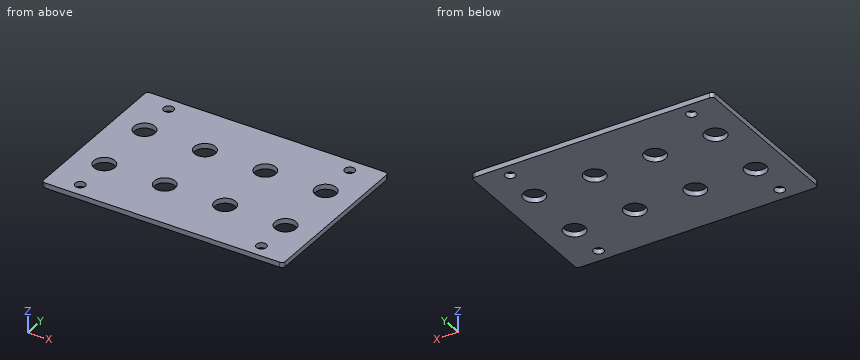
Autodesk Fusion 360 part; units mm, degrees
sketch "Sketch1" plane through (0, 0, 0) normal (0, 0, 1) x (1, 0, 0)
  circle A0 centre (9, 34.525) radius 3.95
  circle A1 centre (9, 15.475) radius 3.95
  line L0 (9, 34.525) -> (9, 15.475) construction
  circle A2 centre (9, 45.975) radius 1.5
  circle A3 centre (9, 4.025) radius 1.5
  line L1 (-1.2896, 25) -> (19.2896, 25) construction
  line L2 (9, 45.975) -> (9, 4.025) construction
  line L3 (5.7, 40.3994) -> (5.7, 10.52)
  line L4 (5.7, 10.52) -> (12.3, 10.52) construction
  line L5 (12.3, 10.52) -> (12.3, 40.3994)
  line L6 (12.3, 40.3994) -> (5.7, 40.3994) construction
  line L7 (5.05, 34.525) -> (12.95, 34.525) construction
  circle A4 centre (27, 34.525) radius 3.95
  line L8 (23.7, 40.3994) -> (23.7, 10.52)
  line L9 (30.3, 10.52) -> (30.3, 40.3994)
  circle A5 centre (27, 15.475) radius 3.95
  circle A6 centre (27, 4.025) radius 1.5
  circle A7 centre (27, 45.975) radius 1.5
  circle A8 centre (45, 34.525) radius 3.95
  line L10 (41.7, 40.3994) -> (41.7, 10.52)
  line L11 (48.3, 10.52) -> (48.3, 40.3994)
  circle A9 centre (45, 15.475) radius 3.95
  circle A10 centre (45, 4.025) radius 1.5
  circle A11 centre (45, 45.975) radius 1.5
  line L12 (0, 50) -> (72, 50)
  line L13 (72, 50) -> (72, 0)
  line L14 (72, 0) -> (0, 0)
  line L15 (0, 0) -> (0, 50)
  line L16 (27, 45.975) -> (27, 4.025) construction
  line L17 (45, 45.975) -> (45, 4.025) construction
  circle A12 centre (63, 34.525) radius 3.95
  line L18 (59.7, 40.3994) -> (59.7, 10.52)
  line L19 (66.3, 10.52) -> (66.3, 40.3994)
  circle A13 centre (63, 15.475) radius 3.95
  circle A14 centre (63, 4.025) radius 1.5
  circle A15 centre (63, 45.975) radius 1.5
  line L20 (63, 45.975) -> (63, 4.025) construction
  line L21 (36, 50) -> (36, 0) construction
  line L22 (0, 25) -> (72, 25) construction
  line L23 (9, 15.475) -> (27, 15.475) construction
  line L24 (18, 15.475) -> (18, 27.912) construction
  point P0 (9, 5.525)
  point P1 (9, 11.525)
  point P2 (27, 34.525)
  point P3 (27, 15.475)
  point P4 (45, 34.525)
  point P5 (45, 15.475)
  point P6 (63, 34.525)
  point P7 (63, 15.475)
  point P8 (45, -15.475)
  point P9 (0, -50)
  point P10 (0, -25)
  point P11 (45, -45.975)
  point P12 (45, -34.525)
  point P13 (0, 50)
  dimension "d4" = 7.9
  dimension "d5" = 7.9
  dimension "d6" = 19.05
  dimension "d7" = 6
  dimension "d8" = 3
  dimension "d9" = 0.65
  dimension "d12" = 18
  dimension "d13" = 0
  dimension "d19" = 50
  dimension "d24" = 41.95
  dimension "d34" = 9
  dimension "d35" = 9
  dimension "d36" = 9
extrude "Extrude1" add sketch "Sketch1" along normal blind 1.5 contours A0 L5 | A0 A1 L3 L5 | A0 L3 | A1 L5 | A1 L3 | A4 L9 | A4 L8 L9 A5 | A4 L8 | L9 A5 | L8 A5 | A6 | A7 | A8 L11 | A8 L10 L11 A9 | A8 L10 | L11 A9 | L10 A9 | A10 | A11 | L12 L13 L14 L15 | A12 L19 | A12 L18 L19 A13 | A12 L18 | L19 A13 | L18 A13 makes body 1
sketch "Sketch2" plane through (0, 0, 0) normal (0, 0, -1) x (1, 0, 0)
  circle A0 centre (9, -4.025) radius 1.5
  circle A1 centre (63, -4.025) radius 1.5
  arc A2 (12.3, -13.3042) -> (5.7, -13.3042) centre (9, -15.475) ccw construction
  line L0 (12.3, -13.3042) -> (12.3, -17.6458) construction
  arc A3 (5.7, -17.6458) -> (12.3, -17.6458) centre (9, -15.475) ccw construction
  line L1 (5.7, -17.6458) -> (5.7, -13.3042) construction
  line L2 (30.3, -13.3042) -> (30.3, -17.6458) construction
  arc A4 (23.7, -17.6458) -> (30.3, -17.6458) centre (27, -15.475) ccw construction
  line L3 (23.7, -17.6458) -> (23.7, -13.3042) construction
  arc A5 (30.3, -13.3042) -> (23.7, -13.3042) centre (27, -15.475) ccw construction
  circle A6 centre (63, -45.975) radius 1.5
  line L4 (48.3, -13.3042) -> (48.3, -17.6458) construction
  arc A7 (41.7, -17.6458) -> (48.3, -17.6458) centre (45, -15.475) ccw construction
  line L5 (41.7, -17.6458) -> (41.7, -13.3042) construction
  arc A8 (48.3, -13.3042) -> (41.7, -13.3042) centre (45, -15.475) ccw construction
  circle A9 centre (9, -45.975) radius 1.5
  line L6 (66.3, -13.3042) -> (66.3, -17.6458) construction
  arc A10 (59.7, -17.6458) -> (66.3, -17.6458) centre (63, -15.475) ccw construction
  line L7 (59.7, -17.6458) -> (59.7, -13.3042) construction
  arc A11 (66.3, -13.3042) -> (59.7, -13.3042) centre (63, -15.475) ccw construction
  line L8 (72, 0) -> (0, 0)
  line L9 (0, 0) -> (0, -50)
  line L10 (0, -50) -> (72, -50)
  line L11 (72, -50) -> (72, 0)
  line L12 (0.4311, -10.2537) -> (71.5689, -10.2537)
  line L13 (71.5689, -10.2537) -> (71.5689, -39.7463)
  line L14 (71.5689, -39.7463) -> (0.4311, -39.7463)
  line L15 (0.4311, -39.7463) -> (0.4311, -10.2537)
  line L16 (0, -25) -> (72, -25) construction
  line L17 (27, -45.975) -> (27, -4.025) construction
  line L18 (45, -45.975) -> (45, -4.025) construction
  line L19 (63, -45.975) -> (63, -4.025) construction
  line L20 (9, -45.975) -> (9, -4.025) construction
  line L21 (36, 0) -> (36, -50) construction
  line L22 (73.0689, -8.7537) -> (73.0689, -41.2463)
  line L23 (73.0689, -41.2463) -> (-1.0689, -41.2463)
  line L24 (-1.0689, -41.2463) -> (-1.0689, -8.7537)
  line L25 (-1.0689, -8.7537) -> (73.0689, -8.7537)
  arc A12 (12.3, -32.3542) -> (5.7, -32.3542) centre (9, -34.525) ccw
  line L26 (12.3, -32.3542) -> (12.3, -36.6958)
  arc A13 (5.7, -36.6958) -> (12.3, -36.6958) centre (9, -34.525) ccw
  line L27 (5.7, -36.6958) -> (5.7, -32.3542)
  arc A14 (66.3, -32.3542) -> (59.7, -32.3542) centre (63, -34.525) ccw
  line L28 (66.3, -32.3542) -> (66.3, -36.6958)
  arc A15 (59.7, -36.6958) -> (66.3, -36.6958) centre (63, -34.525) ccw
  line L29 (59.7, -36.6958) -> (59.7, -32.3542)
  arc A16 (30.3, -32.3542) -> (23.7, -32.3542) centre (27, -34.525) ccw
  line L30 (30.3, -32.3542) -> (30.3, -36.6958)
  arc A17 (23.7, -36.6958) -> (30.3, -36.6958) centre (27, -34.525) ccw
  line L31 (23.7, -36.6958) -> (23.7, -32.3542)
  arc A18 (48.3, -32.3542) -> (41.7, -32.3542) centre (45, -34.525) ccw
  line L32 (48.3, -32.3542) -> (48.3, -36.6958)
  arc A19 (41.7, -36.6958) -> (48.3, -36.6958) centre (45, -34.525) ccw
  line L33 (41.7, -36.6958) -> (41.7, -32.3542)
  dimension "d18" = -1.5
sketch "Sketch3" plane through (0, 0, 0) normal (0, 0, 1) x (1, 0, 0)
  line L0 (0, 50) -> (72, 50)
  line L1 (72, 50) -> (72, 0)
  line L2 (72, 0) -> (0, 0)
  line L3 (0, 0) -> (0, 50)
  circle A0 centre (9, 45.975) radius 1.5
  circle A1 centre (9, 4.025) radius 1.5
  circle A2 centre (9, 34.525) radius 3.15
  circle A3 centre (9, 15.475) radius 3.15
  circle A4 centre (27, 34.525) radius 3.15
  circle A5 centre (27, 45.975) radius 1.5
  circle A6 centre (27, 15.475) radius 3.15
  circle A7 centre (27, 4.025) radius 1.5
  circle A8 centre (45, 34.525) radius 3.15
  circle A9 centre (45, 45.975) radius 1.5
  circle A10 centre (45, 15.475) radius 3.15
  circle A11 centre (45, 4.025) radius 1.5
  circle A12 centre (63, 34.525) radius 3.15
  circle A13 centre (63, 45.975) radius 1.5
  circle A14 centre (63, 15.475) radius 3.15
  circle A15 centre (63, 4.025) radius 1.5
  point P0 (0, 50)
  point P1 (72, 0)
  point P2 (9, 45.975)
  point P3 (9, 4.025)
  point P4 (9, 34.525)
  point P5 (9, 15.475)
  point P6 (27, 15.475)
  point P7 (27, 4.025)
  point P8 (45, 15.475)
  point P9 (45, 4.025)
  point P10 (63, 15.475)
  point P11 (63, 4.025)
  dimension "d25" = 6.3
  dimension "d26" = 6.3
  dimension "d29" = 18
  dimension "d30" = 0
extrude "Extrude3" add sketch "Sketch3" along normal blind 1.5 separate body contours L0 L1 L2 L3 | A5 | A7 | A9 | A11 makes body 2
fillet "Fillet1" radius 1 4 edges at (72, 0, 0.75) (0, 0, 0.75) (72, 50, 0.75) (0, 50, 0.75) on bodies 2
hidden bodies 1
equation "banana_d = 7.9 mm"
equation "ctr_to_ctr = 0.75 in"
equation "flat_inset = 0.65 mm"
equation "d4 = banana_d"
equation "d5 = banana_d"
equation "d6 = ctr_to_ctr"
equation "d7 = 5 mm + 1 mm"
equation "d9 = flat_inset"
equation "x_spacing = 18 mm"
equation "d26 = d25"
equation "d29 = x_spacing"
equation "d36 = d35"
The listing builds one solid part. Answer for the finished solid, in the listing's coordinates (mm). Round coordinates to 2 decimals unless told otherwise and drop trailing zeros. Order: outer loops, then holes, each group sorted by start corner. A loop starts at its lowest first (then second) coordinate and runs counter-clockwise, first axis right, second up. Notation, with made-up numbers: (66.25, 47) -> (73.25, 47) arc R10 cw to (73.25, 53) -> close; hole circle Ø11 at (39, -2). An arc over 180 degrees is marked (long way). Answer as CSV lines item,"result".
Q1. Consider line 1 (Y direction, x = 45, z = 0.7) (3 decimals); line 2 (Y direction, x = 63, z = 0.3) (3 decimals); line 3 (Y direction, x = 65, z = 0.5). Determine where each line is inside the solid, lowest interval first. Write a range as from..to.
Computed values:
line 1,"y = 0..12.325, 18.625..31.375, 37.675..50"
line 2,"y = 0..2.525, 5.525..12.325, 18.625..31.375, 37.675..44.475, 47.475..50"
line 3,"y = 0..13.04, 17.91..32.09, 36.96..50"
Q2. A cutting plane is placed at B-B on x = 63. Determine the outline of the cut face in (y, z) (3 decimals), plus the area to 3 significant figures.
Computed values:
outline,"(0, 0) -> (2.525, 0) -> (2.525, 1.5) -> (0, 1.5) -> close; (5.525, 0) -> (12.325, 0) -> (12.325, 1.5) -> (5.525, 1.5) -> close; (18.625, 0) -> (31.375, 0) -> (31.375, 1.5) -> (18.625, 1.5) -> close; (37.675, 0) -> (44.475, 0) -> (44.475, 1.5) -> (37.675, 1.5) -> close; (47.475, 0) -> (50, 0) -> (50, 1.5) -> (47.475, 1.5) -> close"
area,"47.1 mm^2"
Q3. Given pin 1 (4 mm diameter, centred on x = 63, y = 45.975, fed in from -Z), flat-ended and moving along its own axis, determine where the tip first touches the part or whether it passes through.
Computed values:
pin 1,"stops at z = 0"
Q4. A cutting plane is placed at C-C on z = 1.05. Give the number of separate pieces and of enclosed holes in the cut face, plus the area to 3 significant figures.
Computed values:
separate pieces,"1"
enclosed holes,"12"
area,"3,320 mm^2"
Q5. A cutting plane is placed at A-A on x = 45. Determine the outline of the cut face in (y, z) (3 decimals).
Computed values:
outline,"(0, 0) -> (12.325, 0) -> (12.325, 1.5) -> (0, 1.5) -> close; (18.625, 0) -> (31.375, 0) -> (31.375, 1.5) -> (18.625, 1.5) -> close; (37.675, 0) -> (50, 0) -> (50, 1.5) -> (37.675, 1.5) -> close"
